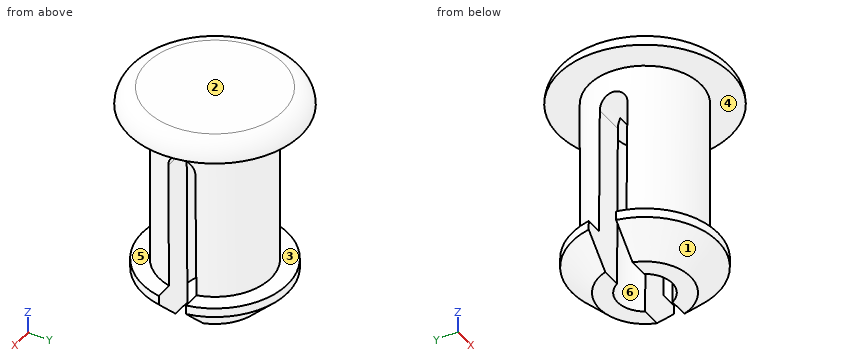
```python
from build123d import *

# Parameters (mm, degrees)
F0_R           = 3.075
F1_DEPTH       = 9
F2_R           = 4.75
F2_R_2         = 3.075
F3_DEPTH       = 1
F4_R           = 0.99999
F5_R           = 4
F5_R_2         = 3.075
F6_DEPTH       = 2
F7_SIZE        = 1.5
F8_R           = 1.5
F9_DEPTH       = 9.5
F11_DEPTH      = 25
F11_DEPTH_BACK = 25


# Not quite as in the source:
# - a fillet or chamfer is up to 0.001 mm smaller than in the source, because OpenCascade refuses the exact size


with BuildPart() as f1:
    # F0 (on Top) → F1 (new body)
    with BuildSketch(Plane.XY):
        Circle(F0_R)
    extrude(amount=F1_DEPTH)

    # F2 (on face) → F3 (join)
    with BuildSketch(Plane.XY.offset(9)):
        Circle(F2_R)
        Circle(F2_R_2, mode=Mode.SUBTRACT)
        Circle(F2_R_2)
    extrude(amount=F3_DEPTH)

    # F4 (radius 1 in the source; OpenCascade refuses exactly that, so slightly less here)
    f4_edges = [f1.edges().sort_by_distance(p)[0] for p in [
        (-4.75, 0, 10),
    ]]
    fillet(f4_edges, radius=F4_R)

    # F5 (on face) → F6 (join)
    with BuildSketch(Plane(origin=(0, 0, 0), x_dir=(1, 0, 0), z_dir=(0, 0, -1))):
        Circle(F5_R)
        Circle(F5_R_2, mode=Mode.SUBTRACT)
        Circle(F5_R_2)
    extrude(amount=F6_DEPTH)

    # F7
    f7_edges = [f1.edges().sort_by_distance(p)[0] for p in [
        (-4, 0, -2),
    ]]
    chamfer(f7_edges, length=F7_SIZE)

    # F8 (on face) → F9 (cut)
    with BuildSketch(Plane(origin=(0, 0, -2), x_dir=(1, 0, 0), z_dir=(0, 0, -1))):
        Circle(F8_R)
    extrude(amount=-F9_DEPTH, mode=Mode.SUBTRACT)

    # F10 (on Right) → F11 (cut, two sides)
    with BuildSketch(Plane.YZ) as f11_sk:
        with BuildLine():
            Line((-0.7, -7), (0.8, -7))
            Line((0.8, -7), (0.7, 7))
            ThreePointArc((0.7, 7), (-0.05, 7.7553762753), (-0.8, 7))
            Line((-0.8, 7), (-0.7, -7))
        make_face()
    extrude(amount=F11_DEPTH, mode=Mode.SUBTRACT)
    extrude(f11_sk.sketch, amount=-F11_DEPTH_BACK, mode=Mode.SUBTRACT)


solid = f1.part
```
Could you check a few things on this model? Use its own coordinates, in mm. Face numbers are marked on the shaded views. A direction names the side the tool comes from. Coordinates: 2 decimals unless noted, no trailing zeros. Write each loop counter-clockwise with the first axis right and the second up, starting at its lowest first coordinate (ties: lowest second). Pieces come first, ordered by that corner, then holes. Notation, with made-up numbers: (26.25, 51.5) -> (31.25, 51.5) arc R20 cw to (31.25, 69.5) -> close; hole circle Ø10 at (71, 2). An arc over 180 degrees is marked (long way). Return JSON: item names as keys, results as strings.
(1) Imagine slicing it at D-D, the plane x = -3.25. Count the separate pieces of the cut face and the enclosed holes in it, then the cut area to 3 significant figures.
Numbers:
{"separate pieces": "3", "enclosed holes": "0", "area": "9.09 mm2"}
(2) Imagine slicing it at C-C, the plane z = 0.5. Please give me the cut outline in (x, y) (3 decimals).
Numbers:
{"outline": "(-2.983, 0.746) -> (-1.301, 0.746) arc R1.5 cw to (1.301, 0.746) -> (2.983, 0.746) arc R3.075 ccw to start; (-2.981, -0.754) arc R3.075 ccw to (2.981, -0.754) -> (1.297, -0.754) arc R1.5 cw to (-1.297, -0.754) -> close"}
(3) I'm going to push flat-ended pins straight in: pin 1 (3 mm diameter, centred on x = 2, z = -0.5, fed in from +Y); pin 2 (4 mm diameter, centred on x = 1.5, z = 7.5, fed in from -Y). Where does each tip first touch, or does it pass through?
Numbers:
{"pin 1": "stops at y = 3.97", "pin 2": "stops at y = -4.75"}
(4) We'd pull the mould along Z, two halves only. Please class the marked faces 1, 2 and 3: +Z half, -Z half, draft (parallel to the pull), parting line (faces both ways), or undercut.
Numbers:
{"face 1": "-Z half", "face 2": "+Z half", "face 3": "undercut"}
(5) Imagine slicing it at A-A, the plane z = 5. Please give me the cut outline in (x, y) (3 decimals), then the cut area to 3 significant figures.
Numbers:
{"outline": "(-2.991, 0.714) -> (-1.319, 0.714) arc R1.5 cw to (1.319, 0.714) -> (2.991, 0.714) arc R3.075 ccw to start; (-2.973, -0.786) arc R3.075 ccw to (2.973, -0.786) -> (1.278, -0.786) arc R1.5 cw to (-1.278, -0.786) -> close", "area": "17.8 mm2"}
(6) Which directions (+Z, -Z, +X, -X, +Y, -Y) give clear straight access to the entire face, cutting with the end or side of a thin tool? Please do the marked faces 4, 5 and 6.
Numbers:
{"face 4": "none", "face 5": "-Y", "face 6": "-Z"}
(7) I need wall thicknesses on L1, parallel to Y at x = -2, z = 6.75; L2, parallel to Y at x = -1, z = 3; L3, parallel to Y at x = -2.5, z = 9.25. Which ranges of each line are inside material? Lowest first, please.
Numbers:
{"L1": "y = -2.34 to -0.8, 0.7 to 2.34", "L2": "y = -2.91 to -1.12, 1.12 to 2.91", "L3": "y = -4 to 4"}
